Can you work these out from the model? Positions are in its coordinate system, mm. A direction names the side the tool comes from. Round coordinates to 2 decimals unless told otherwise and drop trailing zeros. Loops run counter-clockwise (first coordinate to the right, second up) from the corner with the lowest first, then second, coordinate; pieces in that order, holes last. Notation, with made-up numbers: (-35.5, 83.5) -> (-19.5, 83.5) arc R23 cw to (-19.5, 108.5) -> close; hole circle Ø7 at (-12.5, 68.25). An arc over 180 degrees is marked (long way). Use a Markdown table: item, result.
from build123d import *

# Parameters (mm, degrees)
ESQUISSE1_R             = 5
BASE_EXTRUSION_DEPTH    = 6
ESQUISSE2_R             = 6
BOSS_EXTRU_1_DEPTH      = 54
ESQUISSE3_R             = 5
BOSS_EXTRU_2_DEPTH      = 10
CHANFREIN1_SIZE         = 0.5
ENL_V_MAT_EXTRU_1_DEPTH = 1.5


with BuildPart() as part:
    # Esquisse1 → Base-Extrusion (new body)
    with BuildSketch(Plane.XY):
        with Locations(Location((0, 0, 0), (0, 0, 180))):
            Circle(ESQUISSE1_R)
    extrude(amount=BASE_EXTRUSION_DEPTH)

    # Esquisse2 → Boss.-Extru.1 (add)
    with BuildSketch(Plane.XY.offset(6)):
        with Locations(Location((0, 0, 0), (0, 0, 104.477512186))):
            Circle(ESQUISSE2_R)
    extrude(amount=BOSS_EXTRU_1_DEPTH)

    # Esquisse3 → Boss.-Extru.2 (add)
    with BuildSketch(Plane.XY.offset(60)):
        with Locations(Location((0, 0, 0), (0, 0, 180))):
            Circle(ESQUISSE3_R)
    extrude(amount=BOSS_EXTRU_2_DEPTH)

    # Chanfrein1
    chanfrein1_edges = [part.edges().sort_by_distance(p)[0] for p in [
        (1.5, -5.809475019, 6),
        (1.5, -5.809475019, 60),
        (5, 0, 0),
        (5, 0, 70),
    ]]
    chamfer(chanfrein1_edges, length=CHANFREIN1_SIZE)

    # Esquisse5 → Enlèv. mat.-Extru.1 (cut, symmetric)
    with BuildSketch(Plane(origin=(0, 0, 0), x_dir=(0, 0, -1), z_dir=(1, 0, 0))):
        with BuildLine():
            Line((-60, 5), (-53, 5))
            ThreePointArc((-53, 5), (-49.464466094, 13.535533906), (-58, 10))
            Line((-58, 10), (-60, 10))
            Line((-60, 10), (-60, 5))
        make_face()
    extrude(amount=ENL_V_MAT_EXTRU_1_DEPTH, both=True, mode=Mode.SUBTRACT)


solid = part.part
1. Will these pins go through, and if not, where does the flat tip stop? pin 1 Ø1.5 at (y, z) = (2.5, 24.5) entering from -X; pin 2 Ø0.9 at (x, z) = (0.5, 57) entering from +Y; pin 3 Ø1 at (y, z) = (-3.5, 41) entering from +X.
Answer sheet:
| item | result |
|---|---|
| pin 1 | stops at x = -5.74 |
| pin 2 | stops at y = 5 |
| pin 3 | stops at x = 5.2 |
2. I need wall thicknesses on line 1 (X direction, y = 5.25, z = 57); line 2 (X direction, y = 0.25, z = 28); line 3 (X direction, y = 1.25, z = 29). Which ranges of each line are inside material? Lowest first, please.
Answer sheet:
| item | result |
|---|---|
| line 1 | x = -2.9 to -1.5, 1.5 to 2.9 |
| line 2 | x = -5.99 to 5.99 |
| line 3 | x = -5.87 to 5.87 |
3. I want a section at C-C (z = 51). Please give me the cut outline in (x, y), plus the area to 3 significant figures.
Answer sheet:
| item | result |
|---|---|
| outline | (-1.5, 5.42) -> (-1.5, 5.81) arc R6 ccw (long way) to (1.5, 5.81) -> (1.5, 5.42) -> close |
| area | 112 mm² |
4. I want a section at A-A (y = 0). Please give me the cut outline in (x, z), plus the area to 3 significant figures.
Answer sheet:
| item | result |
|---|---|
| outline | (-6, 6.5) -> (-5.5, 6) -> (-5, 6) -> (-5, 0.5) -> (-4.5, 0) -> (4.5, 0) -> (5, 0.5) -> (5, 6) -> (5.5, 6) -> (6, 6.5) -> (6, 59.5) -> (5.5, 60) -> (5, 60) -> (5, 69.5) -> (4.5, 70) -> (-4.5, 70) -> (-5, 69.5) -> (-5, 60) -> (-5.5, 60) -> (-6, 59.5) -> close |
| area | 807 mm² |
5. If we mould it in two halves opening along X, with no side actions, what happens to faces 1 (the flat face through (0, 0, 70)), 2 (the cylindrical face through (5, 0, 65)), 3 (the flat face through (0, 5, 57))? For each: +X half, -X half, draft (parallel to the pull), parting line (faces both ways), or undercut.
Answer sheet:
| item | result |
|---|---|
| face 1 | draft |
| face 2 | parting line |
| face 3 | undercut |
6. I want a section at B-B (z = 38.5). Please give me the cut outline in (x, y).
Answer sheet:
| item | result |
|---|---|
| outline | circle Ø12 at (0, 0) |
7. Which directions (+Z, -Z, +X, -X, +Y, -Y) give clear straight access to the entire face, cutting with the end or side of a thin tool? Please do faces 4 (the cylindrical face through (0.02, 5.25, 51.44)), 5 (the cylindrical face through (5, 0, 3)), 6 (the flat face through (-1.3, -5, 60)), 7 (the flat face through (0, 0, 0)).
Answer sheet:
| item | result |
|---|---|
| face 4 | +Z, +Y |
| face 5 | -Z |
| face 6 | +Z |
| face 7 | -Z, +X, -X, +Y, -Y |
